Geometry: final body of the model. Coordinates: model frame, mm. A direction names the side the tool comes from. Round coordinates to 2 decimals unless told otherwise and drop trailing zeros. Loops run counter-clockwise (first coordinate to the right, second up) from the corner with the lowest first, then second, coordinate; pieces in that order, holes last. Notation, with made-up numbers: M 67.5,52.25 L 123.5,52.25 A12 ccw 123.5,71.25 Z; hole C -32.5,66.25 d2. An arc over 180 degrees is marked long. Answer as a JSON object with one key per item and string values.
```python
from build123d import *

# Parameters (mm, degrees)
SKETCH1_W           = 63.5
SKETCH1_H           = 12.7
BOSS_EXTRUDE1_DEPTH = 38.1
BOSS_EXTRUDE2_DEPTH = 12.7


with BuildPart() as part:
    # Sketch1 → Boss-Extrude1 (new body)
    with BuildSketch(Plane.XY):
        with Locations((31.75, 6.35)):
            Rectangle(SKETCH1_W, SKETCH1_H)
    extrude(amount=BOSS_EXTRUDE1_DEPTH)

    # Sketch1_4 → Boss-Extrude2 (add)
    with BuildSketch(Plane.XY):
        with BuildLine():
            Line((0, 50.8), (0, 12.7))
            Line((0, 12.7), (63.5, 12.7))
            Line((63.5, 12.7), (63.5, 25.4))
            ThreePointArc((63.5, 25.4), (67.219743879, 34.380256121), (76.2, 38.1))
            Line((76.2, 38.1), (114.3, 38.1))
            ThreePointArc((114.3, 38.1), (88.9, 63.5), (114.3, 88.9))
            Line((114.3, 88.9), (38.1, 88.9))
            ThreePointArc((38.1, 88.9), (11.159231637, 77.740768363), (0, 50.8))
        make_face()
        with BuildLine():
            ThreePointArc((139.7, 63.5), (132.260512242, 81.460512242), (114.3, 88.9))
            Line((114.3, 88.9), (114.3, 76.2))
            ThreePointArc((114.3, 76.2), (123.280256121, 72.480256121), (127, 63.5))
            ThreePointArc((127, 63.5), (123.280256121, 54.519743879), (114.3, 50.8))
            Line((114.3, 50.8), (114.3, 38.1))
            ThreePointArc((114.3, 38.1), (132.260512242, 45.539487758), (139.7, 63.5))
        make_face()
        with BuildLine():
            Line((114.3, 76.2), (114.3, 88.9))
            ThreePointArc((114.3, 88.9), (88.9, 63.5), (114.3, 38.1))
            Line((114.3, 38.1), (114.3, 50.8))
            ThreePointArc((114.3, 50.8), (101.6, 63.5), (114.3, 76.2))
        make_face()
    extrude(amount=BOSS_EXTRUDE2_DEPTH)


solid = part.part
```
1) Line query: probe 1 along Y at (x, z) = (29.5, 27.5); probe 2 along Y at (x, z) = (101, 10). Output: solid intervals per line, ascending.
Geometry results:
{"probe 1": "0 to 12.7", "probe 2": "38.1 to 88.9"}
2) Cut plane A-A on z = 9.5. Return the cut outline in (x, y).
Geometry results:
{"outline": "M 0,0 L 63.5,0 L 63.5,25.4 A12.7 cw 76.2,38.1 L 114.3,38.1 A25.4 ccw 114.3,88.9 L 38.1,88.9 A38.1 ccw 0,50.8 Z; hole C 114.3,63.5 d25.4"}
3) Cut plane B-B on x = 124. Return the cut outline in (y, z), and give its area (3 significant figures).
Geometry results:
{"outline": "M 40.03,0 L 55.3,0 L 55.3,12.7 L 40.03,12.7 Z; M 71.7,0 L 86.97,0 L 86.97,12.7 L 71.7,12.7 Z", "area": "388 mm2"}
4) Set-up query: faces 1 (the face through (31, 0, 19)), 2 (the face through (31, 12.7, 25)), 3 (the face through (63.5, 10, 15)). Return all of +Z, -Z, +X, -X, +Y, -Y with unobstructed straight access to the full face (end or side cutting, diameter ignored); none if empty.
Geometry results:
{"face 1": "+Z, -Z, +X, -X, -Y", "face 2": "+Z, +X, -X, +Y", "face 3": "+Z, -Z, +X, -Y"}
5) Cut plane D-D on x = 58. Return the cut outline in (y, z), and give its area (3 significant figures).
Geometry results:
{"outline": "M 0,0 L 88.9,0 L 88.9,12.7 L 12.7,12.7 L 12.7,38.1 L 0,38.1 Z", "area": "1,450 mm2"}
6) First-contact query: pin 1 (4 mm diameter, centred on y = 67, z = 16.5, fed in from +X); pin 2 (5 mm diameter, centred on y = 70, z = 6.5, fed in from -X) (3 decimals); pin 3 (23 mm diameter, centred on x = 51.5, y = 53.5, fed in from +Z); pin 4 (4 mm diameter, centred on x = 102, z = 9.5, fed in from -Y). Flat tips, straight axial feed; report the tip coordinate or a pass-through.
Geometry results:
{"pin 1": "through", "pin 2": "x = 3.855", "pin 3": "z = 12.7", "pin 4": "y = 38.1"}
7) Cut plane C-C on y = 70. Return the cut outline in (x, z), and give its area (3 significant figures).
Geometry results:
{"outline": "M 5.19,0 L 103.39,0 L 103.39,12.7 L 5.19,12.7 Z; M 125.21,0 L 138.85,0 L 138.85,12.7 L 125.21,12.7 Z", "area": "1,420 mm2"}
